Source: CAD feature listing. Evaluate the final solid. Frame: model axes, mm. Face numbers are marked on the shaded views. A direction names the side the tool comes from. Round coordinates to 2 decimals unless told otherwise and drop trailing zeros. Order: outer loops, then holes, each group sorted by start corner. A loop starts at its lowest first (then second) coordinate and runs counter-clockwise, first axis right, second up. Notation, with made-up numbers: (16.25, 24) - (63.25, 24) arc R20 ccw to (63.25, 55) - close; hole circle Ø11 at (-29, 2). An arc over 180 degrees is marked (long way). Put each result on its own line as item: value. Start each with the question number.
1) Line query: probe 1 along X at (y, z) = (-20, 5.5); probe 2 along Y at (x, z) = (16, 3); probe 3 along Y at (x, z) = (0, 4.25) (3 decimals). Output: solid intervals per line, ascending. Write a range as [from, to].
2) Section A-A on y = 0. Output: boundary loops of the cut face in (x, z) (3 decimals), then the cut area to 3 significant figures.
3) Section B-B on x = -25. Output: boundary loops of the cut face in (y, z), then the cut area to 3 significant figures.
4) Contact query for a flat-ended pin moving along its axis: P1, Ø1.5, axis at y = 1.5, z = 4, coming from the -X side. Output: stop coordinate, or through.
5) Section D-D on x = -3. Output: boundary loops of the cut face in (y, z), then the cut area to 3 significant figures.
6) Access query for the marked faces 5, 6 and 7. Directions: +Z, -Z, +X, -X, +Y, -Y. A direction counts if a zero-diameter tool reaches every point of the face in a straight line with its end or side. Return the directions, or none.
7) Section C-C on z = 1. State how many separate pieces and enclosed holes the cut face has, then the cut area to 3 significant figures.
8) Mould query, pull axis Y, two halves, no side actions, for the marked faces 1, 2, 3 and 4. Classes: +Y half, -Y half, draft (parallel to the pull), parting line (faces both ways), or undercut.
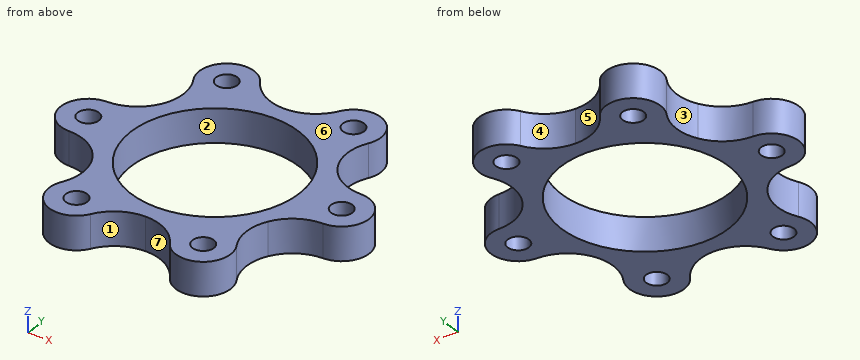
Autodesk Inventor part; units mm, degrees
ref_plane "YZ Plane" through (0, 0, 0) normal (1, 0, 0) x (0, 1, 0)
ref_plane "XZ Plane" through (0, 0, 0) normal (0, 1, 0) x (-1, 0, 0)
ref_plane "XY Plane" through (0, 0, 0) normal (0, 0, 1) x (1, 0, 0)
sketch "Sketch1" plane through (0, 0, 0) normal (0, 0, 1) x (1, 0, 0)
  circle A0 centre (0, 0) radius 19.05
  circle A1 centre (23.8125, 0) radius 2.0193
  arc A2 (23.8832, -5.1938) -> (23.8832, 5.1938) centre (23.8125, 0) ccw
  arc A3 (16.4978, 9.525) -> (23.8832, 5.1938) centre (24.001, 13.857) ccw
  arc A4 (23.8832, -5.1938) -> (16.4978, -9.525) centre (24.001, -13.857) ccw
  circle A5 centre (11.9063, 20.6222) radius 2.0193
  arc A6 (16.4396, 18.0865) -> (7.4436, 23.2803) centre (11.9063, 20.6222) ccw
  arc A7 (0, 19.05) -> (7.4436, 23.2803) centre (0, 27.714) ccw
  arc A8 (16.4396, 18.0865) -> (16.4978, 9.525) centre (24.001, 13.857) ccw
  circle A9 centre (-11.9062, 20.6222) radius 2.0193
  arc A10 (-7.4436, 23.2803) -> (-16.4396, 18.0865) centre (-11.9062, 20.6222) ccw
  arc A11 (-16.4978, 9.525) -> (-16.4396, 18.0865) centre (-24.001, 13.857) ccw
  arc A12 (-7.4436, 23.2803) -> (0, 19.05) centre (0, 27.714) ccw
  circle A13 centre (-23.8125, 0) radius 2.0193
  arc A14 (-23.8832, 5.1938) -> (-23.8832, -5.1938) centre (-23.8125, 0) ccw
  arc A15 (-16.4978, -9.525) -> (-23.8832, -5.1938) centre (-24.001, -13.857) ccw
  arc A16 (-23.8832, 5.1938) -> (-16.4978, 9.525) centre (-24.001, 13.857) ccw
  circle A17 centre (-11.9063, -20.6222) radius 2.0193
  arc A18 (-16.4396, -18.0865) -> (-7.4436, -23.2803) centre (-11.9063, -20.6222) ccw
  arc A19 (0, -19.05) -> (-7.4436, -23.2803) centre (0, -27.714) ccw
  arc A20 (-16.4396, -18.0865) -> (-16.4978, -9.525) centre (-24.001, -13.857) ccw
  circle A21 centre (11.9062, -20.6222) radius 2.0193
  arc A22 (7.4436, -23.2803) -> (16.4396, -18.0865) centre (11.9062, -20.6222) ccw
  arc A23 (16.4978, -9.525) -> (16.4396, -18.0865) centre (24.001, -13.857) ccw
  arc A24 (7.4436, -23.2803) -> (0, -19.05) centre (0, -27.714) ccw
  circle A25 centre (0, 0) radius 15.875
  dimension "d0" = 38.1
  dimension "d1" = 4.0386
  dimension "d2" = 3.175
  dimension "d3" = 23.8125
  dimension "d4" = 8.664
  dimension "d7" = 360
  dimension "d9" = 31.75
extrude "Extrusion1" add sketch "Sketch1" along normal blind 6.35 contours A0 | A0 A3 A2 A4
pattern_circular "Circular Pattern1" count 6 over 360 about axis through (0, 0, 0) along (0, 0, 1) of "Extrusion1"
properties part number "Standardized Plate Spacer" material "Aluminum 6061"
Answer sheet:
1. probe 1: [-17.06, -13.83], [-9.99, -3.94], [3.94, 9.99], [13.83, 17.06]
1. probe 2: [-23.82, -17.18], [-10.53, 10.53], [17.18, 23.82]
1. probe 3: [-19.05, -15.875], [15.875, 19.05]
2. outline: (-29.007, 0) - (-25.832, 0) - (-25.832, 6.35) - (-29.007, 6.35) - close; (-21.793, 0) - (-15.875, 0) - (-15.875, 6.35) - (-21.793, 6.35) - close; (15.875, 0) - (21.793, 0) - (21.793, 6.35) - (15.875, 6.35) - close; (25.832, 0) - (29.007, 0) - (29.007, 6.35) - (25.832, 6.35) - close
2. area: 115 mm^2
3. outline: (-5.06, 0) - (-1.63, 0) - (-1.63, 6.35) - (-5.06, 6.35) - close; (1.63, 0) - (5.06, 0) - (5.06, 6.35) - (1.63, 6.35) - close
3. area: 43.5 mm^2
4. P1: x = -28.95
5. outline: (-19.59, 0) - (-15.59, 0) - (-15.59, 6.35) - (-19.59, 6.35) - close; (15.59, 0) - (19.59, 0) - (19.59, 6.35) - (15.59, 6.35) - close
5. area: 50.8 mm^2
6. face 5: +Z, -Z, +Y
6. face 6: +Z, +X, -X, +Y, -Y
6. face 7: +Z, -Z, -Y
7. separate pieces: 1
7. enclosed holes: 7
7. area: 898 mm^2
8. face 1: -Y half
8. face 2: undercut
8. face 3: undercut
8. face 4: +Y half
